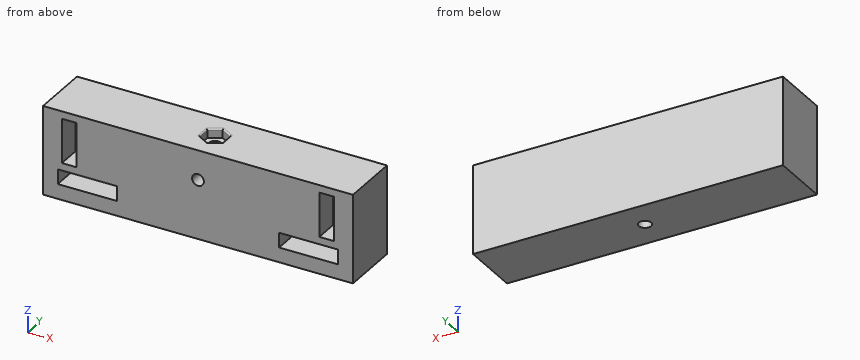
from build123d import *

# Parameters (mm, degrees)
ESQUISSE1_W             = 105
ESQUISSE1_H             = 20
BOSS_EXTRU_1_DEPTH      = 30
ENL_V_MAT_EXTRU_1_DEPTH = 3
CONG_2_R                = 0.5
ESQUISSE8_R             = 2.103774153
ENL_V_MAT_EXTRU_3_DEPTH = 112.018016556
ESQUISSE9_R             = 2
ENL_V_MAT_EXTRU_5_DEPTH = 5
ESQUISSE10_W            = 20
ESQUISSE10_H            = 5
ESQUISSE10_W_2          = 5
ESQUISSE10_H_2          = 15
ENL_V_MAT_EXTRU_6_DEPTH = 8


with BuildPart() as part:
    # Esquisse1 → Boss.-Extru.1 (new body)
    with BuildSketch(Plane.XY):
        with Locations((-52.5, 10)):
            Rectangle(ESQUISSE1_W, ESQUISSE1_H)
    extrude(amount=BOSS_EXTRU_1_DEPTH)

    # Esquisse2 → Enlèv. mat.-Extru.1 (cut)
    with BuildSketch(Plane.XY.offset(30)):
        Polygon((-52.5, 5.4966679), (-48.6, 7.74833395), (-48.6, 12.25166605), (-52.5, 14.5033321), (-56.4, 12.25166605), (-56.4, 7.74833395), align=None)
    extrude(amount=-ENL_V_MAT_EXTRU_1_DEPTH, mode=Mode.SUBTRACT)

    # Congé2
    cong_2_edges = [part.edges().sort_by_distance(p)[0] for p in [
        (-54.45, 6.622500925, 30),
        (-50.55, 6.622500925, 30),
        (-48.6, 10, 30),
        (-50.55, 13.377499075, 30),
        (-54.45, 13.377499075, 30),
        (-56.4, 10, 30),
    ]]
    fillet(cong_2_edges, radius=CONG_2_R)

    # Esquisse8 → Enlèv. mat.-Extru.3 (cut, through all)
    with BuildSketch(Plane.XY):
        with Locations((-52.5, 10)):
            Circle(ESQUISSE8_R)
    extrude(amount=ENL_V_MAT_EXTRU_3_DEPTH, mode=Mode.SUBTRACT)

    # Esquisse9 → Enlèv. mat.-Extru.5 (cut)
    with BuildSketch(Plane.XZ):
        with Locations((-52.5, 20)):
            Circle(ESQUISSE9_R)
    extrude(amount=-ENL_V_MAT_EXTRU_5_DEPTH, mode=Mode.SUBTRACT)

    # Esquisse10 → Enlèv. mat.-Extru.6 (cut)
    with BuildSketch(Plane.XZ):
        with Locations((-15, 7.5)):
            Rectangle(ESQUISSE10_W, ESQUISSE10_H)
        with Locations((-8.89, 20)):
            Rectangle(ESQUISSE10_W_2, ESQUISSE10_H_2)
        with Locations((-96.11, 20)):
            Rectangle(ESQUISSE10_W_2, ESQUISSE10_H_2)
        with Locations((-90, 7.5)):
            Rectangle(ESQUISSE10_W, ESQUISSE10_H)
    extrude(amount=-ENL_V_MAT_EXTRU_6_DEPTH, mode=Mode.SUBTRACT)


solid = part.part
Work out the finished part from the listing and answer in its coordinate system (mm). Round coordinates to 2 decimals unless told otherwise and drop trailing zeros. Loops run counter-clockwise (first coordinate to the right, second up) from the corner with the lowest first, then second, coordinate; pieces in that order, holes last. Notation, with made-up numbers: (38.5, 1.25) -> (87.5, 1.25) arc R11 cw to (87.5, 14.25) -> close; hole circle Ø5 at (-21, 30). An arc over 180 degrees is marked (long way). Use one line per item in the form item = value.
(1) Flat-ended cylindrical pins translate along their axes: P1, Ø1.5, axis at x = -96, z = 19.5, coming from the -Y side; P2, Ø3.5, axis at x = -52.5, y = 10, coming from the -Z side; P3, Ø4, axis at x = -52, y = 8.5, coming from the +Z side. Find the tip coordinate at first contact, or state that the pin passes through.
Answer list:
P1 = 8
P2 = through
P3 = 27
(2) Find section D-D on z = 7.25. Give the vertices of the cut face in (x, y).
Answer list:
outline = (-105, 0) -> (-100, 0) -> (-100, 8) -> (-80, 8) -> (-80, 0) -> (-25, 0) -> (-25, 8) -> (-5, 8) -> (-5, 0) -> (0, 0) -> (0, 20) -> (-105, 20) -> close; hole circle Ø4.21 at (-52.5, 10)
(3) Find section B-B on x = -7.5. Give the vertices of the cut face in (y, z), then the cut area to 3 significant figures.
Answer list:
outline = (0, 0) -> (20, 0) -> (20, 30) -> (0, 30) -> (0, 27.5) -> (8, 27.5) -> (8, 12.5) -> (0, 12.5) -> (0, 10) -> (8, 10) -> (8, 5) -> (0, 5) -> close
area = 440 mm2
(4) Find section A-A on z = 14. Give the vertices of the cut face in (x, y).
Answer list:
outline = (-105, 0) -> (-98.61, 0) -> (-98.61, 8) -> (-93.61, 8) -> (-93.61, 0) -> (-11.39, 0) -> (-11.39, 8) -> (-6.39, 8) -> (-6.39, 0) -> (0, 0) -> (0, 20) -> (-105, 20) -> close; hole circle Ø4.21 at (-52.5, 10)
(5) Straight lines are drawn through the part: line 1 (X direction, y = 5.75, z = 21.5); line 2 (Z direction, x = -97, y = 4.25); line 3 (Y direction, x = -52.5, z = 18.75). For each, find the intervals that lie inside material, in ascending order.
Answer list:
line_1 = -105 to -98.61, -93.61 to -11.39, -6.39 to 0
line_2 = 0 to 5, 10 to 12.5, 27.5 to 30
line_3 = 5 to 7.9, 12.1 to 20
(6) Find section C-C on z = 20. Give the vertices of the cut face in (x, y).
Answer list:
outline = (-105, 0) -> (-98.61, 0) -> (-98.61, 8) -> (-93.61, 8) -> (-93.61, 0) -> (-54.5, 0) -> (-54.5, 5) -> (-50.5, 5) -> (-50.5, 0) -> (-11.39, 0) -> (-11.39, 8) -> (-6.39, 8) -> (-6.39, 0) -> (0, 0) -> (0, 20) -> (-105, 20) -> close; hole circle Ø4.21 at (-52.5, 10)
